```python
from build123d import *

# Parameters (mm, degrees)
SKETCH_1_R      = 10
SKETCH_1_R_2    = 5
EXTRUDE_1_DEPTH = 9
EXTRUDE_2_DEPTH = 3
EXTRUDE_3_DEPTH = 3
EXTRUDE_4_DEPTH = 3
SKETCH_5_R      = 2.5
EXTRUDE_5_DEPTH = 5


with BuildPart() as part:
    # 草图1 → 凸台-拉伸1 (new, symmetric)
    with BuildSketch(Plane(origin=(0, 0, 0), x_dir=(0, 0, -1), z_dir=(1, 0, 0))):
        Circle(SKETCH_1_R)
        Circle(SKETCH_1_R_2, mode=Mode.SUBTRACT)
    extrude(amount=EXTRUDE_1_DEPTH, both=True)

    # 草图2 → 凸台-拉伸2 (add, symmetric)
    with BuildSketch(Plane(origin=(0, 0, 0), x_dir=(0, 0, -1), z_dir=(1, 0, 0))):
        with BuildLine():
            Line((9.84807753, -1.736481777), (48.899871085, 12.477208672))
            Line((48.899871085, 12.477208672), (126.133884246, 48.492020479))
            Line((126.133884246, 48.492020479), (121.907701629, 57.555098349))
            Line((121.907701629, 57.555098349), (45.069390993, 21.72480566))
            Line((45.069390993, 21.72480566), (6.427876097, 7.660444431))
            ThreePointArc((6.427876097, 7.660444431), (9.396926208, 3.420201433), (9.84807753, -1.736481777))
        make_face()
    extrude(amount=EXTRUDE_2_DEPTH, both=True)

    # 草图3 → 凸台-拉伸3 (add, symmetric)
    with BuildSketch(Plane(origin=(0, 0, 0), x_dir=(0, 0, -1), z_dir=(1, 0, 0))):
        with BuildLine():
            Line((-9.760845357, -2.173913043), (-4.880422678, -24.086956522))
            ThreePointArc((-4.880422678, -24.086956522), (0, -28), (4.880422678, -24.086956522))
            Line((4.880422678, -24.086956522), (9.760845357, -2.173913043))
            ThreePointArc((9.760845357, -2.173913043), (0, -10), (-9.760845357, -2.173913043))
        make_face()
    extrude(amount=EXTRUDE_3_DEPTH, both=True)

    # 草图4 → 凸台-拉伸4 (add, symmetric)
    with BuildSketch(Plane(origin=(0, 0, 0), x_dir=(0, 0, -1), z_dir=(1, 0, 0))):
        with BuildLine():
            Line((9.760845357, -2.173913043), (9.26353243, -4.406842549))
            ThreePointArc((9.26353243, -4.406842549), (10.386363512, -2.195237961), (12.433854391, -0.795335967))
            Line((12.433854391, -0.795335967), (9.84807753, -1.736481777))
            ThreePointArc((9.84807753, -1.736481777), (9.806900669, -1.955683838), (9.760845357, -2.173913043))
        make_face()
    extrude(amount=EXTRUDE_4_DEPTH, both=True)

    # 草图5 → 凸台-拉伸5 (add)
    with BuildSketch(Plane(origin=(0, 56.973055831, -122.179112512), x_dir=(-1, 0, 0), z_dir=(0, 0.422618261740695, -0.9063077870366522))):
        with Locations(Location((0, -4.357787137, 0), (0, 0, 90))):
            Circle(SKETCH_5_R)
    extrude(amount=EXTRUDE_5_DEPTH)


solid = part.part
```
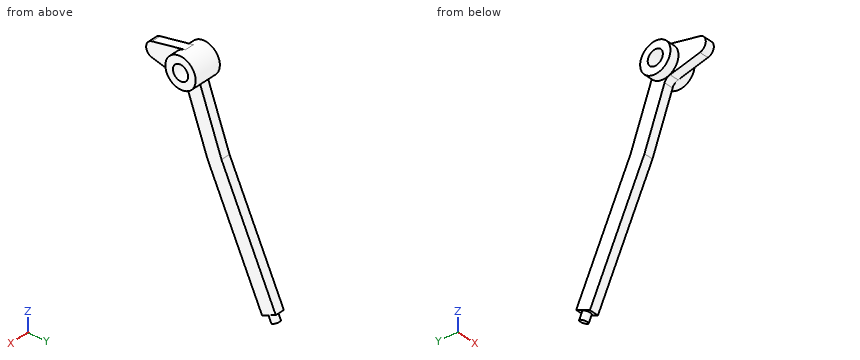
Geometry check sheet. Reference: the model listing, model coordinates, mm. Round coordinates to 2 decimals unless told otherwise and drop trailing zeros. Order: outer loops, then holes, each group sorted by start corner. A loop starts at its lowest first (then second) coordinate and runs counter-clockwise, first axis right, second up. Notation, with made-up numbers: (35, -19.5) - (71, -19.5) arc R6 cw to (71, -15.5) - close; hole circle Ø7 at (52.25, 86.5). An arc over 180 degrees is marked (long way). Use a Markdown table: item, result. Add a question column.
(1) Sectioned sample at B-B, the plane x = -6. Enter the section's corners in (y, z).
(2) Depth check by flat-ended pin: pin 1 (6 mm diameter, centred on x = 5.5, y = -18, fed in from +Z); pin 2 (10 mm diameter, centred on x = -7, z = -66.5, fed in from -Y). Enter the tip coordinate at first touch or a pass-through.
(3) Sectioned sample at C-C, the plane y = 44. Enter the section's corners in (x, z), and give its area (3 significant figures).
(4) Sectioned sample at A-A, the plane z = 0. Enter the section's corners in (x, y).
(5) Material ranges on line 1 along Y through (x, z) = (-2.5, 0); line 2 along Y through (x, z) = (5.75, 0); line 3 along X through (y, z) = (37, -79), recorded low to high. Write a range as [from, to].
Answers below:
| question | item | result |
|---|---|---|
| 1 | outline | circle Ø20 at (0, 0); hole circle Ø10 at (0, 0) |
| 2 | pin 1 | z = 6.61 |
| 2 | pin 2 | y = 19.29 |
| 3 | outline | (-3, -116.5) - (3, -116.5) - (3, -92.84) - (-3, -92.84) - close |
| 3 | area | 142 mm² |
| 4 | outline | (-9, -10) - (-3, -10) - (-3, -28) - (3, -28) - (3, -10) - (9, -10) - (9, -5) - (-9, -5) - close; (-9, 5) - (9, 5) - (9, 10) - (-9, 10) - close |
| 5 | line 1 | [-28, -5], [5, 10] |
| 5 | line 2 | [-10, -5], [5, 10] |
| 5 | line 3 | [-3, 3] |
